```python
from build123d import *

# Parameters (mm, degrees)
SKETCH1_R           = 1.375
BOSS_EXTRUDE1_DEPTH = 3
FILLET1_R           = 4


with BuildPart() as part:
    # Sketch1 → Boss-Extrude1 (new body)
    with BuildSketch(Plane.XY):
        with BuildLine():
            Line((-4.5, -0.8), (-4.5, 9))
            ThreePointArc((-4.5, 9), (-2.171359962, 12.941471288), (2.404531518, 12.803712421))
            ThreePointArc((2.404531518, 12.803712421), (9.257380419, 11.803998346), (14.585878733, 16.227579703))
            ThreePointArc((14.585878733, 16.227579703), (14.895094025, 17.089921688), (15, 18))
            Line((15, 18), (15, 30))
            Line((15, 30), (23, 30))
            Line((23, 30), (23.968058833, 13.771849702))
            ThreePointArc((23.968058833, 13.771849702), (19.101398678, 0.356849969), (6, -5.3))
            Line((6, -5.3), (0, -5.3))
            ThreePointArc((0, -5.3), (-3.181980515, -3.981980515), (-4.5, -0.8))
        make_face()
        Circle(SKETCH1_R, mode=Mode.SUBTRACT)
        with Locations((0, 9)):
            Circle(SKETCH1_R, mode=Mode.SUBTRACT)
        with Locations((20, 14)):
            Circle(SKETCH1_R, mode=Mode.SUBTRACT)
    extrude(amount=BOSS_EXTRUDE1_DEPTH)

    # Fillet1
    fillet1_edges = [part.edges().sort_by_distance(p)[0] for p in [
        (15, 30, 1.5),
        (23, 30, 1.5),
    ]]
    fillet(fillet1_edges, radius=FILLET1_R)


solid = part.part
```
Design review of the part built by this model. Coordinates are the model's own, in mm. A direction names the side the tool comes from. Round coordinates to 2 decimals unless told otherwise and drop trailing zeros. Order: outer loops, then holes, each group sorted by start corner. A loop starts at its lowest first (then second) coordinate and runs counter-clockwise, first axis right, second up. Notation, with made-up numbers: (-11, 4.5) - (22, 4.5) arc R13 ccw to (22, 18.5) - close; hole circle Ø9 at (-25, 12.5). An arc over 180 degrees is marked (long way). Return JSON: item names as keys, results as strings.
Q1. Consider section B-B on y = 12. Write out the cut boundary in (x, z), plus the area to 3 significant figures.
Computed values:
{"outline": "(-3.35, 0) - (4.04, 0) - (4.04, 3) - (-3.35, 3) - close; (9.87, 0) - (23.99, 0) - (23.99, 3) - (9.87, 3) - close", "area": "64.5 mm2"}
Q2. Machinability: for faces 4 (the flat face through (15, 22, 1)), 5 (the flat face through (13, 9, 0)), which of the approach directions +Z, -Z, +X, -X, +Y, -Y give a long, thin tool a straight path to every point of the face, cutting with its end or side? Answer none if there is none.
Computed values:
{"face 4": "+Z, -Z, -X, +Y", "face 5": "-Z, +X, -X, +Y, -Y"}
Q3. Consider section C-C on x = -1. Write out the cut boundary in (y, z).
Computed values:
{"outline": "(-5.19, 0) - (-0.94, 0) - (-0.94, 3) - (-5.19, 3) - close; (0.94, 0) - (8.06, 0) - (8.06, 3) - (0.94, 3) - close; (9.94, 0) - (13.39, 0) - (13.39, 3) - (9.94, 3) - close"}
Q4. Consider section D-D on z = 2.6. Give the number of separate pieces and of enclosed holes in the cut face, plus the area to 3 significant figures.
Computed values:
{"separate pieces": "1", "enclosed holes": "3", "area": "562 mm2"}
Q5. The part is to be moulded in two halves that separate along X. For faces 1 (the flat face through (-4.5, 4, 1)), 2 (the flat face through (13, 9, 3)), 3 (the cylindrical face through (-0.179, 10.363, 1.479)), say which applies: pulls with the +X half, pulls with the -X half, needs draft (parallel to the pull), parting line crosses it, or undercut.
Computed values:
{"face 1": "pulls with the -X half", "face 2": "needs draft", "face 3": "undercut"}
Q6. Consider section A-A on x = 20. Write out the cut boundary in (y, z) (3 decimals).
Computed values:
{"outline": "(1.386, 0) - (12.625, 0) - (12.625, 3) - (1.386, 3) - close; (15.375, 0) - (29.925, 0) - (29.925, 3) - (15.375, 3) - close"}
Q7. Wall thickness on L1, parallel to Y at x = 0, z = 1.05 (3 decimals); L2, parallel to Y at x = 20, z = 1.15 (3 decimals); L3, parallel to Y at x = 16.75, z = 2: over which ranges is each line inside the solid? List them lowest first. Write a range as [from, to].
Computed values:
{"L1": "y = [-5.3, -1.375], [1.375, 7.625], [10.375, 13.5]", "L2": "y = [1.386, 12.625], [15.375, 29.925]", "L3": "y = [-1.74, 29.31]"}
